```python
from build123d import *

# Parameters (mm, degrees)
BOSS_EXTRUDE1_DEPTH = 3
SKETCH4_W           = 2.9
SKETCH4_H           = 20
CUT_EXTRUDE1_DEPTH  = 4


with BuildPart() as part:
    # Sketch3 → Boss-Extrude1 (new body)
    with BuildSketch(Plane(origin=(0, 0, 0), x_dir=(0.999999536, -0.000963417, 0), z_dir=(0, 0, 1))):
        Polygon((87.907726379, 95.819824151), (-72.092273621, 95.665677408), (-72.092273621, 49.448943998), (87.95225233, 49.603133638), align=None)
    extrude(amount=BOSS_EXTRUDE1_DEPTH)

    # Sketch4 → Cut-Extrude1 (cut, through all)
    with BuildSketch(Plane.XY.offset(3)):
        with Locations((1.5, 73.735087911)):
            Rectangle(SKETCH4_W, SKETCH4_H)
        with Locations((11.5, 73.735087911)):
            Rectangle(SKETCH4_W, SKETCH4_H)
        with Locations((71.5, 73.735087911)):
            Rectangle(SKETCH4_W, SKETCH4_H)
        with Locations((81.5, 73.735087911)):
            Rectangle(SKETCH4_W, SKETCH4_H)
    extrude(amount=-CUT_EXTRUDE1_DEPTH, mode=Mode.SUBTRACT)


solid = part.part
```
Model file for the job. Use its own axes, mm. A direction names the side the tool comes from. Coordinates: 2 decimals unless noted, no trailing zeros. Write each loop counter-clockwise with the first axis right and the second up, starting at its lowest first coordinate (ties: lowest second). Pieces come first, ordered by that corner, then holes. Notation, with made-up numbers: (-40, 80.5) - (-2, 80.5) arc R28 ccw to (-2, 116.5) - close; hole circle Ø2 at (53.25, -17). An arc over 180 degrees is marked (long way). One line per item, written item: value. Start each with the question number.
1. Slice it at C-C (y = 67). Write the cut outline in (x, z).
2. Slice it at B-B (z = 1.7). Write the cut outline in (x, y).
3. Tool access for faces 1 (the flat face through (7, 73, 0)), 2 (the flat face through (81, 83.735, 2)): list every direction of +Z, -Z, +X, -X, +Y, -Y with a clear straight run to the whole face (end or side of a thin tool).
4. Slice it at A-A (y = 80). Write the cut outline in (x, z), plus the area to 3 significant figures.
5. Mould opens along Y. For faces 3 (the flat face through (9, 95.735, 1)), 4 (the flat face through (70.05, 74, 2)), 5 (the flat face through (7, 49.518, 1)) say: released by +Y, released by -Y, zero draft, split by the parting line, or undercut.
6. Flat gauge pin, fed straight in: pin 1 (0.9 mm diameter, centred on y = 76, z = 1, fed in from -X). Where does the tip first touch, or does it go through?
7. Probe line 1 (X direction, y = 73.5, z = 2.1); line 2 (X direction, y = 91, z = 2.2). List the from-to ranges inside material, lowest first. Write a range as from..to.
Answers below:
1. outline: (-72.03, 0) - (0.05, 0) - (0.05, 3) - (-72.03, 3) - close; (2.95, 0) - (10.05, 0) - (10.05, 3) - (2.95, 3) - close; (12.95, 0) - (70.05, 0) - (70.05, 3) - (12.95, 3) - close; (72.95, 0) - (80.05, 0) - (80.05, 3) - (72.95, 3) - close; (82.95, 0) - (88, 0) - (88, 3) - (82.95, 3) - close
2. outline: (-72.04, 49.52) - (88, 49.52) - (88, 95.74) - (-72, 95.74) - close; hole (0.05, 63.74) - (2.95, 63.74) - (2.95, 83.74) - (0.05, 83.74) - close; hole (10.05, 63.74) - (12.95, 63.74) - (12.95, 83.74) - (10.05, 83.74) - close; hole (70.05, 63.74) - (72.95, 63.74) - (72.95, 83.74) - (70.05, 83.74) - close; hole (80.05, 63.74) - (82.95, 63.74) - (82.95, 83.74) - (80.05, 83.74) - close
3. face 1: -Z, +X, -X, +Y, -Y
3. face 2: +Z, -Z
4. outline: (-72.02, 0) - (0.05, 0) - (0.05, 3) - (-72.02, 3) - close; (2.95, 0) - (10.05, 0) - (10.05, 3) - (2.95, 3) - close; (12.95, 0) - (70.05, 0) - (70.05, 3) - (12.95, 3) - close; (72.95, 0) - (80.05, 0) - (80.05, 3) - (72.95, 3) - close; (82.95, 0) - (88, 0) - (88, 3) - (82.95, 3) - close
4. area: 445 mm^2
5. face 3: released by +Y
5. face 4: undercut
5. face 5: released by -Y
6. pin 1: stops at x = -72.02
7. line 1: x = -72.02..0.05, 2.95..10.05, 12.95..70.05, 72.95..80.05, 82.95..88
7. line 2: x = -72..88
